Print and shaded views of the part. All mm, measured from the part's lowest x, y and z. A direction names the side the tool comes from. Round coordinates to 2 decimals unless told otherwise and drop trailing zeros. Loops run counter-clockwise (first coordinate to the right, second up) from the corner with the lowest first, then second, coordinate; pieces in that order, holes last. Notation, with made-up numbers: (22.5, 37.5) -> (38.5, 37.5) arc R28 cw to (38.5, 59.5) -> close; hole circle Ø11 at (-37, -13). An arc over 180 degrees is marked (long way). Answer as CSV lines item,"result".
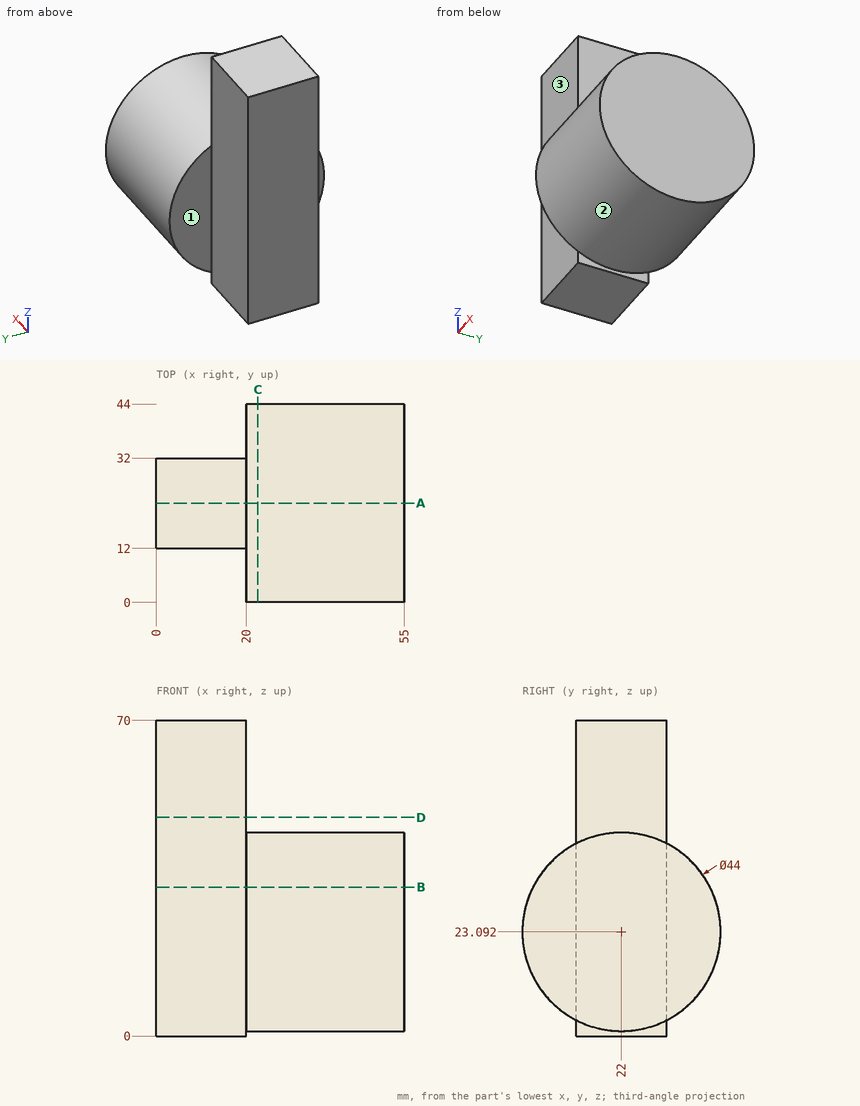
Q1. Slice it at D-D, the plane z = 48.5. Give the cut face in (x, y).
Results:
outline,"(0, 12) -> (20, 12) -> (20, 32) -> (0, 32) -> close"
Q2. Drop flat-ended pins along their axis: pin 1 Ø12 at (x, z) = (39, 10) entering from -Y (1 decimal); pin 2 Ø2 at (x, y) = (40, 36) entering from +Z; pin 3 Ø1.5 at (x, z) = (6, 8) entering from -Y. Give the stop position or say it passes through.
Results:
pin 1,"y = 1.2"
pin 2,"z = 40.84"
pin 3,"y = 12"
Q3. Slice it at B-B, the plane z = 33. Give the cut face in (x, y).
Results:
outline,"(0, 12) -> (20, 12) -> (20, 2.36) -> (55, 2.36) -> (55, 41.64) -> (20, 41.64) -> (20, 32) -> (0, 32) -> close"
Q4. Probe L1, parallel to X at y = 35.5, z = 10; L2, parallel to Y at x = 4.5, z = 63.5; L3, parallel to X at y = 25, z = 55. List the from-to ranges inside material, lowest first. Write a range as [from, to].
Results:
L1,"[20, 55]"
L2,"[12, 32]"
L3,"[0, 20]"
Q5. Slice it at A-A, the plane y = 22. Give the cut face in (x, z), and give its area (3 significant figures).
Results:
outline,"(0, 0) -> (20, 0) -> (20, 1.09) -> (55, 1.09) -> (55, 45.09) -> (20, 45.09) -> (20, 70) -> (0, 70) -> close"
area,"2,940 mm2"
Q6. Tool access for the marked faces 1, 2 and 3: list every direction of +Z, -Z, +X, -X, +Y, -Y with a clear straight run to the whole face (end or side of a thin tool).
Results:
face 1,"+Z, -Z, -X, +Y"
face 2,"+X"
face 3,"+Z, -Z, -X, -Y"
Q7. Slice it at C-C, the plane x = 22.5. Give the cut face in (y, z), and give its area (3 significant figures).
Results:
outline,"circle Ø44 at (22, 23.09)"
area,"1,520 mm2"
